Autodesk Inventor part; units mm, degrees
ref_plane "YZ Plane" through (0, 0, 0) normal (1, 0, 0) x (0, 1, 0)
ref_plane "XZ Plane" through (0, 0, 0) normal (0, 1, 0) x (-1, 0, 0)
ref_plane "XY Plane" through (0, 0, 0) normal (0, 0, 1) x (1, 0, 0)
sketch "Foam Scheme" plane through (0, 0, 0) normal (0, 1, 0) x (-1, 0, 0)
  line L0 (819.5, -94) -> (-819.5, -94)
  line L1 (-819.5, -94) -> (-819.5, 94)
  line L2 (-819.5, 94) -> (819.5, 94)
  line L3 (819.5, 94) -> (819.5, -94)
  circle A0 centre (797.5, -72) radius 9.5
  circle A1 centre (742.5, -72) radius 9.5
  circle A2 centre (687.5, -72) radius 9.5
  circle A3 centre (632.5, -72) radius 9.5
  circle A4 centre (577.5, -72) radius 9.5
  circle A5 centre (522.5, -72) radius 9.5
  circle A6 centre (467.5, -72) radius 9.5
  circle A7 centre (412.5, -72) radius 9.5
  circle A8 centre (357.5, -72) radius 9.5
  circle A9 centre (302.5, -72) radius 9.5
  circle A10 centre (247.5, -72) radius 9.5
  circle A11 centre (192.5, -72) radius 9.5
  circle A12 centre (137.5, -72) radius 9.5
  circle A13 centre (82.5, -72) radius 9.5
  circle A14 centre (27.5, -72) radius 9.5
  circle A15 centre (-27.5, -72) radius 9.5
  circle A16 centre (-82.5, -72) radius 9.5
  circle A17 centre (-137.5, -72) radius 9.5
  circle A18 centre (797.5, 72) radius 9.5
  circle A19 centre (742.5, 72) radius 9.5
  circle A20 centre (687.5, 72) radius 9.5
  circle A21 centre (632.5, 72) radius 9.5
  circle A22 centre (577.5, 72) radius 9.5
  circle A23 centre (522.5, 72) radius 9.5
  circle A24 centre (467.5, 72) radius 9.5
  circle A25 centre (412.5, 72) radius 9.5
  circle A26 centre (357.5, 72) radius 9.5
  circle A27 centre (302.5, 72) radius 9.5
  circle A28 centre (247.5, 72) radius 9.5
  circle A29 centre (192.5, 72) radius 9.5
  circle A30 centre (137.5, 72) radius 9.5
  circle A31 centre (82.5, 72) radius 9.5
  circle A32 centre (27.5, 72) radius 9.5
  circle A33 centre (-27.5, 72) radius 9.5
  circle A34 centre (-82.5, 72) radius 9.5
  circle A35 centre (-137.5, 72) radius 9.5
  circle A36 centre (-192.5, -72) radius 9.5
  circle A37 centre (-192.5, 72) radius 9.5
  circle A38 centre (-247.5, -72) radius 9.5
  circle A39 centre (-247.5, 72) radius 9.5
  circle A40 centre (-302.5, -72) radius 9.5
  circle A41 centre (-302.5, 72) radius 9.5
  circle A42 centre (-357.5, -72) radius 9.5
  circle A43 centre (-357.5, 72) radius 9.5
  circle A44 centre (-412.5, -72) radius 9.5
  circle A45 centre (-412.5, 72) radius 9.5
  circle A46 centre (-467.5, -72) radius 9.5
  circle A47 centre (-467.5, 72) radius 9.5
  circle A48 centre (-522.5, -72) radius 9.5
  circle A49 centre (-522.5, 72) radius 9.5
  circle A50 centre (-577.5, -72) radius 9.5
  circle A51 centre (-577.5, 72) radius 9.5
  circle A52 centre (-632.5, -72) radius 9.5
  circle A53 centre (-632.5, 72) radius 9.5
  circle A54 centre (-687.5, -72) radius 9.5
  circle A55 centre (-687.5, 72) radius 9.5
  circle A56 centre (-742.5, -72) radius 9.5
  circle A57 centre (-742.5, 72) radius 9.5
  circle A58 centre (-797.5, -72) radius 9.5
  circle A59 centre (-797.5, 72) radius 9.5
  point P0 (0, 0)
  dimension "d0" = 1639
  dimension "d1" = 819.5
  dimension "d2" = 188
  dimension "d3" = 94
  dimension "d4" = 19
  dimension "d5" = 22
  dimension "d6" = 22
  dimension "d9" = 55
  dimension "d12" = 144
extrude "Foam Body" add sketch "Foam Scheme" along normal blind 1.5
properties part number "Foam NPS 16" material "Rubber, Silicone"
The listing builds one solid part. Answer for the finished solid, in the listing's coordinates (mm). Round coordinates to 2 decimals unless told otherwise and drop trailing zeros. Put each result on its own line as item: value. Start each with the question number.
(1) Find section A-A (y = 0.55). State how many separate pieces and enclosed holes the cut face has, plus the area to 3 significant figures.
(2) Given P1, Ø11.5, axis at x = -522.5, z = -72, coming from the +Y side, flat-ended and moving along its own axis, determine where the tip first touches the part or whether it passes through.
(3) Straight lines are drawn through the part: probe 1 along Z at (x, y) = (192.5, 0.6); probe 2 along Z at (x, y) = (139, 1.1). For each, find the intervals that lie inside material, in ascending order. Write a range as from..to.
Reply:
1. separate pieces: 1
1. enclosed holes: 60
1. area: 291,000 mm^2
2. P1: through
3. probe 1: -94..-81.5, -62.5..62.5, 81.5..94
3. probe 2: -94..-81.38, -62.62..62.62, 81.38..94
